from build123d import *

# Parameters (mm, degrees)
F1_DEPTH = 3
F5_SIZE2 = 0.803838
F5_SIZE  = 2.99999
F4_W     = 7
F4_H     = 2.8
F6_DEPTH = 12.5


# Not quite as in the source:
# - a fillet or chamfer is up to 0.001 mm smaller than in the source, because OpenCascade refuses the exact size


with BuildPart() as f1:
    # F0 (on Top) → F1 (new body)
    with BuildSketch(Plane.XY):
        with BuildLine():
            Line((4, 0), (92.5, 0))
            ThreePointArc((92.5, 0), (94.267766953, 0.732233047), (95, 2.5))
            Line((95, 2.5), (95, 6.6861086512))
            ThreePointArc((95, 6.6861086512), (94.6715622153, 7.784234218), (93.7941202395, 8.5216938563))
            Line((93.7941202395, 8.5216938563), (41.5145959947, 31.1391284496))
            ThreePointArc((41.5145959947, 31.1391284496), (33.9924781689, 31.3092893749), (28.4809169267, 26.1873850415))
            Line((28.4809169267, 26.1873850415), (20, 8))
            Line((20, 8), (8, 8))
            Line((8, 8), (9.0498639623, 20))
            Line((9.0498639623, 20), (6, 20))
            ThreePointArc((6, 20), (1.7573593129, 18.2426406871), (0, 14))
            Line((0, 14), (0, 4))
            ThreePointArc((0, 4), (1.1715728753, 1.1715728753), (4, 0))
        make_face()
    extrude(amount=F1_DEPTH)

    # F5 (size 3 and 0.8038475773 in the source; OpenCascade refuses exactly that, so slightly less here)
    f5_edges = [f1.edges().sort_by_distance(p)[0] for p in [
        (8.524932, 14, 3),
    ]]
    f5_side = f1.faces().sort_by_distance((8.524932, 14, 1.5))[0]
    chamfer(f5_edges, length=F5_SIZE, length2=F5_SIZE2, reference=f5_side)

    # F4 (on line) → F6 (cut, symmetric)
    with BuildSketch(Plane(origin=(61.5, 0, 35.5070415552), x_dir=(0, 1, 0), z_dir=(0.8660254038, 0, 0.5))):
        with Locations((3.5, -39.6)):
            Rectangle(F4_W, F4_H)
    extrude(amount=F6_DEPTH, both=True, mode=Mode.SUBTRACT)


solid = f1.part
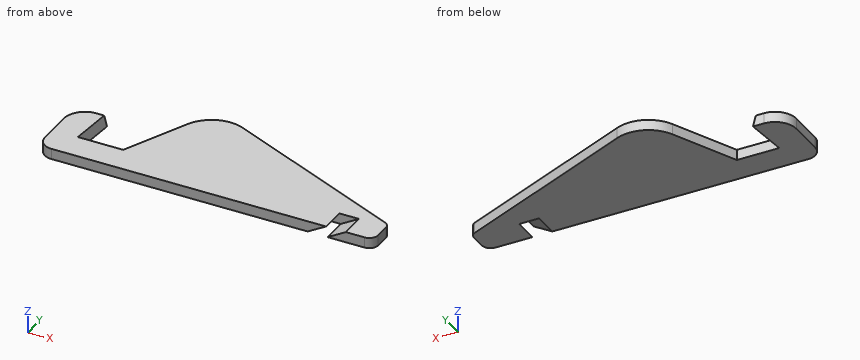
Work out the finished part from the listing and answer in its coordinate system (mm). Round coordinates to 2 decimals unless told otherwise and drop trailing zeros. Write each loop counter-clockwise with the first axis right and the second up, starting at its lowest first coordinate (ties: lowest second). Pieces come first, ordered by that corner, then holes. Notation, with made-up numbers: (70.25, 34.25) -> (115.25, 34.25) arc R30 cw to (115.25, 60.25) -> close; hole circle Ø2 at (-21, 58). An arc over 180 degrees is marked (long way). Write each question's results on one line, items separated by ' | '.
Item 1: A cutting plane is placed at B-B, the plane z = 0.7. Determine the outline of the cut face in (x, y).
Result set:
outline: (0, 4) arc R4 ccw to (4, 0) -> (77.61, 0) -> (77.61, 7) -> (83.21, 7) -> (83.21, 0) -> (92.5, 0) arc R2.5 ccw to (95, 2.5) -> (95, 6.69) arc R2 ccw to (93.79, 8.52) -> (41.51, 31.14) arc R10 ccw to (28.48, 26.19) -> (20, 8) -> (7.81, 8) -> (8.86, 20) -> (6, 20) arc R6 ccw to (0, 14) -> close
Item 2: Find the intervals of material crossed by line 1 along X through (y, z) = (4.5, 2.4); line 2 along X through (y, z) = (13, 0.25); line 3 along Y through (x, z) = (28.5, 2), in increasing order. Write a range as [from, to].
Result set:
line 1: [0, 80.56], [86.16, 95] | line 2: [0, 8.37], [22.33, 83.44] | line 3: [0, 26.23]
Item 3: A cutting plane is placed at C-C, the plane x = 52. Determine the outline of the cut face in (y, z).
Result set:
outline: (0, 0) -> (26.6, 0) -> (26.6, 3) -> (0, 3) -> close
Item 4: Flat-ended cylindrical pins translate along their axes: P1, Ø1.5, axis at x = 82, z = 1.5, coming from the -Y side; P2, Ø1.5, axis at y = 16.5, z = 2, coming from the -X side; P3, Ø0.9, axis at x = 7, z = 1.5, coming from the +Y side. Find the tip coordinate at first contact, or state that the pin passes through.
Result set:
P1: y = 7 | P2: x = 0.26 | P3: y = 20
